Autodesk Inventor part; units mm, degrees
ref_plane "Start plane" through (0, 0, -20) normal (0, 0, 1) x (1, 0, 0)
ref_plane "End plane" through (0, 0, 880) normal (0, 0, 1) x (1, 0, 0)
ref_plane "Work Plane4" through (0, 20, -20) normal (0, -0.7071, -0.7071) x (1, 0, 0)
ref_plane "Start plane" through (0, 0, -20) normal (0, 0, 1) x (1, 0, 0)
ref_plane "End plane" through (0, 0, 880) normal (0, 0, 1) x (1, 0, 0)
sketch "Sketch" plane through (0, 0, 0) normal (0, 0, 1) x (1, 0, 0)
  line L0 (-20, -12) -> (-20, 12)
  line L1 (-12, 20) -> (12, 20)
  line L2 (20, 12) -> (20, -12)
  line L3 (12, -20) -> (-12, -20)
  arc A0 (-20, -12) -> (-12, -20) centre (-12, -12) ccw
  arc A1 (-12, 20) -> (-20, 12) centre (-12, 12) ccw
  arc A2 (20, 12) -> (12, 20) centre (12, 12) ccw
  arc A3 (12, -20) -> (20, -12) centre (12, -12) ccw
  arc A4 (-12, 16) -> (-16, 12) centre (-12, 12) ccw
  line L4 (-12, 16) -> (12, 16)
  arc A5 (16, 12) -> (12, 16) centre (12, 12) ccw
  line L5 (16, 12) -> (16, -12)
  arc A6 (12, -16) -> (16, -12) centre (12, -12) ccw
  line L6 (12, -16) -> (-12, -16)
  arc A7 (-16, -12) -> (-12, -16) centre (-12, -12) ccw
  line L7 (-16, -12) -> (-16, 12)
  line L8 (0, 30.3196) -> (0, -30.3196) construction
  line L9 (-30.3196, 0) -> (30.3196, 0) construction
  dimension "d7" = 8
  dimension "d10" = 40
  dimension "d11" = 40
  dimension "d12" = 4
  dimension "d15" = 20
  dimension "d16" = 20
extrude "Body" add sketch "Sketch" along normal up to surface (900 mm away) from surface at -20
sketch "Sketch3" plane through (0, 0, 0) normal (0, 0, 1) x (1, 0, 0)
  line L0 (0, 0) -> (10, 0)
ref_plane "Work Plane3" through (0, 0, 0) normal (0, -1, 0) x (1, 0, 0)
sketch "Sketch4" plane through (0, 0, 0) normal (0, -1, 0) x (1, 0, 0)
  line L0 (-2, -20) -> (12, -20)
  line L1 (-2, 880) -> (12, 880)
  dimension "d18" = 900
ref_plane "Work Plane4" through (0, 20, -20) normal (0, -0.7071, -0.7071) x (1, 0, 0)
split "Split1" plane through (0, 20, -20) removes the side toward (0, -0.7071, -0.7071)
ref_plane "Work Plane5" through (0, 20, 1520) normal (0, -0.7071, 0.7071) x (1, 0, 0)
split "Split2" plane through (0, 20, 1520) removes the side toward (0, -0.7071, 0.7071)
ref_plane "Work Plane6" through (-1000, 12, 880) normal (0, 0, 1) x (1, 0, 0)
split "Split3" plane through (-1000, 12, 880) removes the side toward (0, 0, 1)
equation "\"d7\" = G_IR"
equation "\"d10\" = G_H"
equation "\"d11\" = G_W"
equation "\"d12\" = G_T"
equation "\"d15\" = 0.5 * d10"
equation "\"d16\" = 0.5 * d11"
equation "\"d3\" = G_L"
equation "\"G_W\" = 40"
equation "\"G_H\" = 40"
equation "\"G_T\" = 4"
equation "\"G_IR\" = 8"
equation "\"G_L\" = d18"
equation "\"G_OFFSET_START\" = 20"
equation "\"G_OFFSET_END\" = -620"
equation "\"d13\" = -G_OFFSET_START"
equation "\"d14\" = G_OFFSET_END + B_L"
properties part number "DIN EN 10219-2 - 40 x 40 x 4  - 900" material "Steel, Mild"
Work out the finished part from the listing and answer in its coordinate system (mm). A direction names the side the tool comes from. Give positions to 0.01 mm unless a question says otherwise; leave off trailing zeros. Loops run counter-clockwise (first coordinate to the right, second up) from the corner with the lowest first, then second, coordinate; pieces in that order, holes last. Notation, with made-up numbers: (-20, 26.5) -> (29, 26.5) arc R26 ccw to (29, 40.5) -> close; hole circle Ø10 at (82.5, -8). An arc over 180 degrees is marked (long way). Use a Markdown table: item, result. Add a question column.
1) Each of these flat-tipped pins is pushed along its axis until it touches: P1, Ø3, axis at x = 15, z = 596.5, coming from the -Y side; P2, Ø5, axis at x = -14.5, y = -8.5, coming from the -Z side. Where does it stop, or does it pass through?
2) For a pull along X with two mould halves and no side action, classify faces 3 (the flat face through (0, 20, 424)), 4 (the flat face through (20, 0, 428)), 5 (the flat face through (0, 16, 426)), 6 (the flat face through (-20, 0, 428)) as +X half, -X half, draft (parallel to the pull), parting line (faces both ways), or undercut.
3) The part is cut by section B-B, the plane x = 1. Determine the outline of the cut face in (y, z).
4) Which of the six approach directions +Z, -Z, +X, -X, +Y, -Y give full straight-line access (tool end or side, diameter ignored) to faces 1 (the flat face through (16, 0, 428)), 2 (the flat face through (-16.4, 0.1, 880))?
5) The part is cut by section A-A, the plane z = 116.5. Determine the outline of the cut face in (x, y), plus the area to 3 significant figures.
6) The part is cut by section C-C, the plane y = -5.5. Determine the outline of the cut face in (x, z), plus the area to 3 significant figures.
7) Consider line 1 along Y through (x, z) = (5.5, 34.5); line 2 along Y through (x, z) = (-13, 264.5). Determine where each line is inside the solid, lowest interval first.
Reported:
| question | item | result |
|---|---|---|
| 1 | P1 | stops at y = -19.86 |
| 1 | P2 | stops at z = 6.5 |
| 2 | face 3 | draft |
| 2 | face 4 | +X half |
| 2 | face 5 | undercut |
| 2 | face 6 | -X half |
| 3 | outline | (-20, 20) -> (-16, 16) -> (-16, 880) -> (-20, 880) -> close; (16, -16) -> (20, -20) -> (20, 880) -> (16, 880) -> close |
| 4 | face 1 | +Z, -Z |
| 4 | face 2 | +Z, +X, -X, +Y, -Y |
| 5 | outline | (-20, -12) arc R8 ccw to (-12, -20) -> (12, -20) arc R8 ccw to (20, -12) -> (20, 12) arc R8 ccw to (12, 20) -> (-12, 20) arc R8 ccw to (-20, 12) -> close; hole (-16, -12) arc R4 ccw to (-12, -16) -> (12, -16) arc R4 ccw to (16, -12) -> (16, 12) arc R4 ccw to (12, 16) -> (-12, 16) arc R4 ccw to (-16, 12) -> close |
| 5 | area | 535 mm^2 |
| 6 | outline | (-20, 5.5) -> (-16, 5.5) -> (-16, 880) -> (-20, 880) -> close; (16, 5.5) -> (20, 5.5) -> (20, 880) -> (16, 880) -> close |
| 6 | area | 7,000 mm^2 |
| 7 | line 1 | y = -20 to -16, 16 to 20 |
| 7 | line 2 | y = -19.94 to -15.87, 15.87 to 19.94 |
